Autodesk Inventor part; units mm, degrees
ref_plane "YZ Plane" through (0, 0, 0) normal (1, 0, 0) x (0, 1, 0)
ref_plane "XZ Plane" through (0, 0, 0) normal (0, 1, 0) x (-1, 0, 0)
ref_plane "XY Plane" through (0, 0, 0) normal (0, 0, 1) x (1, 0, 0)
sketch "Sketch1" plane through (0, 0, 0) normal (0, 1, 0) x (-1, 0, 0)
  circle A0 centre (0, 0) radius 3.2
  line L0 (3.2, 0) -> (-3.2, 0)
  dimension "d0" = 6.4
revolve "Revolution1" add sketch "Sketch1" angle 360 about axis through (-3.2, 0, 0) along (1, 0, 0) picked at (1.0667, -1.9947) contours A0 L0
sketch "Sketch2" plane through (0, 0, 0) normal (1, 0, 0) x (0, 1, 0)
  line L0 (-1.9733, 5.6826) -> (-7.2021, 5.6826)
  line L1 (-7.2021, 5.6826) -> (-7.2021, -6.4165)
  line L2 (-7.2021, -6.4165) -> (-1.9733, -6.4165)
  line L3 (-1.9733, -6.4165) -> (-1.9733, 5.6826)
  line L4 (5.3731, 6.6744) -> (2.8267, 6.6744)
  line L5 (2.8267, 6.6744) -> (2.8267, -5.9008)
  line L6 (2.8267, -5.9008) -> (5.3731, -5.9008)
  line L7 (5.3731, -5.9008) -> (5.3731, 6.6744)
  circle A0 centre (0, 0) radius 3.2
  point P0 (2.8267, -1.5)
  point P1 (2.8267, 1.5)
  dimension "d2" = 4.8
  dimension "d8" = 3
extrude "Extrusion1" cut sketch "Sketch2" along normal mid plane 10 contours L3 A0 L2 L1 L0 | L3 A0 | A0 L5 | L5 L4 L7 L6 A0
sketch "Sketch3" plane through (0, -1.9733, 0) normal (0, -1, 0) x (1, 0, 0)
  circle A0 centre (0, 0) radius 2.5191
  circle A1 centre (0, 0) radius 1.5
  dimension "d5" = 3
extrude "Extrusion2" add sketch "Sketch3" along normal blind 8 contours A1
thread "Thread1"
sketch "Sketch4" plane through (0, 2.8267, 0) normal (0, 1, 0) x (1, 0, 0)
  line L0 (-1.3899, 0) -> (-0.7247, 1.1522)
  line L1 (-0.7247, 1.1522) -> (0.6057, 1.1522)
  line L2 (0.6057, 1.1522) -> (1.2709, 0)
  line L3 (1.2709, 0) -> (0.6057, -1.1522)
  line L4 (0.6057, -1.1522) -> (-0.7247, -1.1522)
  line L5 (-0.7247, -1.1522) -> (-1.3899, 0)
  point P0 (-0.0595, 0)
extrude "Extrusion3" cut sketch "Sketch4" against normal blind 2
properties part number "500-113" material "Aluminum 6061"
For this review, take the finished solid that the model builds, in its own axes (mm). A direction names the side the tool comes from. Coordinates: 2 decimals unless noted, no trailing zeros. Order: outer loops, then holes, each group sorted by start corner. A loop starts at its lowest first (then second) coordinate and runs counter-clockwise, first axis right, second up. Notation, with made-up numbers: (-33.5, -5) -> (-21.5, -5) arc R32 ccw to (-21.5, 21) -> close; hole circle Ø9 at (70.25, -28.5). An arc over 180 degrees is marked (long way). Return JSON: item names as keys, results as strings.
1. We need section A-A on x = 0. Write out the cut boundary in (y, z).
Answer block:
{"outline": "(-9.97, -1.5) -> (-1.97, -1.5) -> (-1.97, -2.52) arc R3.2 ccw to (2.83, -1.5) -> (2.83, -1.15) -> (0.83, -1.15) -> (0.83, 1.15) -> (2.83, 1.15) -> (2.83, 1.5) arc R3.2 ccw to (-1.97, 2.52) -> (-1.97, 1.5) -> (-9.97, 1.5) -> close"}
2. The part is to be moulded in two halves that separate along Z. For faces 3 (the flat face through (0, -1.973, 2)), 4 (the cylindrical face through (-1.5, -5.92, -0.07)), 5 (the flat face through (-1.06, 1.84, -0.57)), say which applies: +Z half, -Z half, draft (parallel to the pull), parting line (faces both ways), or undercut.
Answer block:
{"face 3": "draft", "face 4": "parting line", "face 5": "undercut"}
3. We need section D-D on z = 2.25. Write out the cut boundary in (x, y), and give its area (3 significant figures).
Answer block:
{"outline": "(-1.13, -1.97) -> (1.13, -1.97) arc R2.28 ccw (long way) to start", "area": "15.8 mm²"}
4. For line 1 (Y direction, x = -0.5, z = 1); line 2 (Z direction, x = 0, y = -5.75); line 3 (Z direction, x = -1, y = -2.25), list the stretches that pass through material, from the lowest coordinate up. Write a range as from..to.
Answer block:
{"line 1": "-9.97..0.83", "line 2": "-1.5..1.5", "line 3": "-1.12..1.12"}
5. Machinability: for faces 1 (the flat face through (0, -9.973, 0)), 2 (the flat face through (0, 2, -1.152)), which of the approach directions +Z, -Z, +X, -X, +Y, -Y give a long, thin tool a straight path to every point of the face, cutting with its end or side? Answer none if there is none.
Answer block:
{"face 1": "+Z, -Z, +X, -X, -Y", "face 2": "+Y"}
6. We need section B-B on z = 0.5. Write out the cut boundary in (x, y).
Answer block:
{"outline": "(-2.47, -1.97) -> (-1.41, -1.97) -> (-1.41, -9.97) -> (1.41, -9.97) -> (1.41, -1.97) -> (2.47, -1.97) arc R3.16 ccw to (1.41, 2.83) -> (0.98, 2.83) -> (0.98, 0.83) -> (-1.1, 0.83) -> (-1.1, 2.83) -> (-1.41, 2.83) arc R3.16 ccw to start"}
7. We need section C-C on y = -3.5. Write out the cut boundary in (x, z).
Answer block:
{"outline": "circle Ø3 at (0, 0)"}
8. For pin 1 Ø0.7 at (x, y) = (0, 2) entering from +Z; pin 2 Ø3 at (x, y) = (1.5, -4.5) entering from -Z; pin 3 Ø2.5 at (x, z) = (-0.5, 0) entering from +Y, all flat-tipped, find the tip position at first contact; note any pin that passes through.
Answer block:
{"pin 1": "z = 2.74", "pin 2": "z = -1.5", "pin 3": "y = 2.83"}
